CAD build for the part. Positions are in the model's coordinates, mm. A direction names the side the tool comes from. Give positions to 0.01 mm unless a question says otherwise; leave off trailing zeros. Write each loop counter-clockwise with the first axis right and the second up, starting at its lowest first coordinate (ties: lowest second). Pieces come first, ordered by that corner, then holes. Notation, with made-up numbers: (-14, 75) - (39, 75) arc R31 cw to (39, 102) - close; hole circle Ø2 at (27.25, -14.5). An arc over 180 degrees is marked (long way). Put each result on its own line as item: value. Start each with the question number.
1. Cut at D-D on z = -36. List the corners of the cut face in (x, y) (3 decimals).
2. Drop flat-ended pins along their axis: pin 1 (2 mm diameter, centred on y = 9, z = -26.55, fed in from +X); pin 2 (2 mm diameter, centred on x = 26.5, z = -24.5, fed in from +Y); pin 3 (10 mm diameter, centred on y = -5.5, z = -17.5, fed in from +X); pin 4 (20 mm diameter, centred on x = 33.5, z = -20, fed in from -Y). Give the stop position or say it passes through.
3. Cut at B-B on z = -26.55. List the corners of the cut face in (x, y) (3 decimals), and give its area (3 significant figures).
4. Mould opens along Z. For faces 4 (the flat face through (22, 0, -16)), 5 (the cylindrical face through (10.698, -4.44, -8.874)), 6 (the flat face through (30, 10, -31.5)), 7 (the flat face through (6.675, 12, -27)) say: +Z half, -Z half, draft (parallel to the pull), parting line (faces both ways), or undercut.
5. Wall check: line 1 (X direction, y = 12.5, z = -28) (3 decimals); line 2 (Z direction, x = 24, y = 8.5); line 3 (X direction, y = 16.75, z = -12) (3 decimals). Give the ranges that are in metal, low to high.
6. Cut at C-C on y = -4.5. List the corners of the cut face in (x, z) (3 decimals), and give its area (4 significant figures).
7. Cut at A-A on y = 5. List the corners of the cut face in (x, z) (3 decimals).
8. Tool access for faces 1 (the cylindrical face through (10.698, 5.06, -37.374)), 2 (the flat face through (4.675, 12, -16)), 3 (the cylindrical face through (42.047, 9.793, -6.154)): list every direction of +Z, -Z, +X, -X, +Y, -Y with a clear straight run to the whole face (end or side of a thin tool).
from build123d import *

# Parameters (mm, degrees)
SKETCH1_W           = 45
SKETCH1_H           = 31.5
BOSS_EXTRUDE1_DEPTH = 20
CUT_EXTRUDE1_DEPTH  = 17
SKETCH3_R           = 0.8
CUT_EXTRUDE2_DEPTH  = 5.825
BOSS_EXTRUDE2_START = -7
SKETCH5_W           = 30.5
SKETCH5_H           = 9
SKETCH5_R           = 1.375
SKETCH5_W_2         = 9
SKETCH5_H_2         = 20
BOSS_EXTRUDE2_DEPTH = 7.5


with BuildPart() as part:
    # Sketch1 → Boss-Extrude1 (new body)
    with BuildSketch(Plane(origin=(0, 0, 0), x_dir=(1, 0, 0), z_dir=(0, 1, 0))):
        with Locations((22.5, 15.75)):
            Rectangle(SKETCH1_W, SKETCH1_H)
    extrude(amount=BOSS_EXTRUDE1_DEPTH)

    # Sketch2 → Cut-Extrude1 (cut)
    with BuildSketch(Plane(origin=(0, 20, 0), x_dir=(1, 0, 0), z_dir=(0, 1, 0))):
        Polygon((39.175, 28.5), (6.675, 28.5), (6.675, 25.5), (4.675, 25.5), (4.675, 6), (6.675, 6), (6.675, 3), (39.175, 3), (39.175, 8.2), (40.325, 8.2), (40.325, 23.3), (39.175, 23.3), align=None)
    extrude(amount=-CUT_EXTRUDE1_DEPTH, mode=Mode.SUBTRACT)

    # Sketch3 → Cut-Extrude2 (cut)
    with BuildSketch(Plane.ZY.offset(-39.175)):
        with Locations((-26.55, 9)):
            Circle(SKETCH3_R)
        with Locations((-6.05, 9)):
            Circle(SKETCH3_R)
    extrude(amount=-CUT_EXTRUDE2_DEPTH, mode=Mode.SUBTRACT)

    # Sketch5 → Boss-Extrude2 (add)
    # profile 1 of 2: a face of its own
    with BuildSketch(Plane.ZY.offset(BOSS_EXTRUDE2_START)):
        with Locations((-15.25, -4.5)):
            Rectangle(SKETCH5_W, SKETCH5_H)
        with Locations((-24, -4.5)):
            Circle(SKETCH5_R, mode=Mode.SUBTRACT)
        with Locations((-7.5, -4.5)):
            Circle(SKETCH5_R, mode=Mode.SUBTRACT)
    # profile 2 of 2: a face of its own
    with BuildSketch(Plane.ZY.offset(BOSS_EXTRUDE2_START)):
        with Locations((-36, 10)):
            Rectangle(SKETCH5_W_2, SKETCH5_H_2)
        with Locations((-36, 5)):
            Circle(SKETCH5_R, mode=Mode.SUBTRACT)
        with Locations((-36, 15)):
            Circle(SKETCH5_R, mode=Mode.SUBTRACT)
    extrude(amount=-BOSS_EXTRUDE2_DEPTH)


solid = part.part
Report:
1. outline: (7, 0) - (14.5, 0) - (14.5, 3.625) - (7, 3.625) - close; (7, 6.375) - (14.5, 6.375) - (14.5, 13.625) - (7, 13.625) - close; (7, 16.375) - (14.5, 16.375) - (14.5, 20) - (7, 20) - close
2. pin 1: stops at x = 45
2. pin 2: stops at y = 3
2. pin 3: stops at x = 14.5
2. pin 4: stops at y = 0
3. outline: (0, 0) - (7, 0) - (7, -9) - (14.5, -9) - (14.5, 0) - (45, 0) - (45, 8.2) - (39.175, 8.2) - (39.175, 3) - (6.675, 3) - (6.675, 20) - (0, 20) - close; (39.175, 9.8) - (45, 9.8) - (45, 20) - (39.175, 20) - close
3. area: 406 mm²
4. face 4: draft
4. face 5: undercut
4. face 6: -Z half
4. face 7: undercut
5. line 1: x = 0 to 6.675, 39.175 to 45
5. line 2: z = -31.5 to -28.5, -3 to 0
5. line 3: x = 0 to 4.675, 40.325 to 45
6. outline: (7, -30.5) - (14.5, -30.5) - (14.5, -25.375) - (7, -25.375) - close; (7, -22.625) - (14.5, -22.625) - (14.5, -8.875) - (7, -8.875) - close; (7, -6.125) - (14.5, -6.125) - (14.5, 0) - (7, 0) - close
6. area: 187.5 mm²
7. outline: (0, -31.5) - (7, -31.5) - (7, -34.625) - (14.5, -34.625) - (14.5, -31.5) - (45, -31.5) - (45, 0) - (0, 0) - close; (7, -40.5) - (14.5, -40.5) - (14.5, -37.375) - (7, -37.375) - close; hole (4.675, -25.5) - (6.675, -25.5) - (6.675, -28.5) - (39.175, -28.5) - (39.175, -23.3) - (40.325, -23.3) - (40.325, -8.2) - (39.175, -8.2) - (39.175, -3) - (6.675, -3) - (6.675, -6) - (4.675, -6) - close
8. face 1: +X, -X
8. face 2: +Y
8. face 3: +X
